Read the model definition and answer for the solid it produces. Units are mm, in the model's axes. A direction names the side the tool comes from. Coordinates: 2 decimals unless noted, no trailing zeros. Loops run counter-clockwise (first coordinate to the right, second up) from the corner with the lowest first, then second, coordinate; pieces in that order, holes last. Notation, with made-up numbers: M 77.5,84 L 98.5,84 A23 cw 98.5,93 Z; hole C 10,21.5 d9. An arc over 180 degrees is marked long. Use one line per item in the form item = value. Start each with the question number.
1. Flat-ended cylindrical pins translate along their axes: pin 1 (1.8 mm diameter, centred on x = -4, y = 0.5, fed in from -Z); pin 2 (2 mm diameter, centred on x = -4.5, y = 18.5, fed in from +Z); pin 3 (1.8 mm diameter, centred on x = -5, z = 7.5, fed in from +Y). Find the tip coordinate at first contact, or state that the pin passes through.
2. For a pull along Y with two mould halves and no side action, classify faces 5 (the flat face through (-4, 1, 11.8)), 6 (the flat face through (-4, -17, 2)), 7 (the cylindrical face through (-6.43, 18.9, 1.83)), 8 (the flat face through (-4, 1, 13.8)) as released by +Y, released by -Y, zero draft, split by the parting line, or undercut.
3. The part is cut by section D-D (x = -2.3). Give the vertices of the cut face in (y, z).
4. A tool of negligible diameter and unlimited length cuts with its end or side. For faces 1 (the flat face through (-4, -11, 6)), 2 (the flat face through (-4, 16, 0.7)), 3 (the flat face through (-4, 16, 3)), 4 (the flat face through (-3, -14, 3)), from which of +Z, -Z, +X, -X, +Y, -Y can it reach the whole face along a straight path? Write none if from no direction.
5. The part is cut by section A-A (y = -15). Give the vertices of the cut face in (x, z).
6. The part is cut by section B-B (z = 4.25). Give the vertices of the cut face in (x, y).
7. The part is cut by section C-C (x = -3.95). Give the vertices of the cut face in (y, z), plus the area to 3 significant figures.
8. Find the intervals of material crossed by probe 1 along X at (y, z) = (17.25, 2.25); probe 2 along Y at (x, z) = (-3.95, 1.8); probe 3 along Y at (x, z) = (-6.2, 4), in increasing order. Write a range as [from, to].
Autodesk Inventor part; units mm, degrees
ref_plane "YZ Plane" through (0, 0, 0) normal (1, 0, 0) x (0, 1, 0)
ref_plane "XZ Plane" through (0, 0, 0) normal (0, 1, 0) x (-1, 0, 0)
ref_plane "XY Plane" through (0, 0, 0) normal (0, 0, 1) x (1, 0, 0)
sketch "Sketch1" plane through (0, 0, 0) normal (0, 0, 1) x (1, 0, 0)
  line L0 (-7, -17) -> (7, -17)
  line L1 (-7, -17) -> (-1, -17)
  line L2 (-1, -17) -> (-1, -11)
  line L3 (-1, -11) -> (-7, -11)
  line L4 (-7, -11) -> (-7, -17)
  line L5 (-5, 19.5) -> (-0.9, 19.5)
  line L6 (-0.9, 19.5) -> (-0.9, 13)
  line L7 (-0.9, 13) -> (-7, 13)
  line L8 (-7, 13) -> (-7, 17.5)
  line L9 (-7, 17.5) -> (-7, -20)
  line L10 (-0.9, 13) -> (-7, 13)
  line L11 (-7, 13) -> (-7, 15)
  line L12 (-7, 15) -> (-0.9, 15)
  line L13 (-0.9, 15) -> (-0.9, 13)
  line L14 (-7, -11) -> (-1, -11)
  line L15 (-1, -11) -> (-1, -13)
  line L16 (-1, -13) -> (-7, -13)
  line L17 (-7, -13) -> (-7, -11)
  circle A0 centre (-3.95, 17.25) radius 0.9
  circle A1 centre (-4, -15) radius 0.9
  arc A2 (-5, 19.5) -> (-7, 17.5) centre (-5, 17.5) ccw
  point P0 (0, 0)
  point P1 (0, 0)
  point P2 (-0.9, 15)
  dimension "d0" = 2
extrude "Extrusion1" add sketch "Sketch1" along normal blind 3 contours L4 L16 L2 L0 | L8 A2 L5 L6 L12
extrude "Extrusion2" add sketch "Sketch1" along normal blind 11.8 contours L8 L12 L6 L7 | L4 L3 L2 L16
sketch "Sketch2" plane through (0, 0, 11.8) normal (0, 0, 1) x (1, 0, 0)
  line L0 (-7, 15) -> (-0.9, 15)
  line L1 (-1, -13) -> (-7, -13)
  line L2 (-0.9, 15) -> (-7, 15)
  line L3 (-7, 15) -> (-7, -13)
  line L4 (-7, -13) -> (-0.9, -13)
  line L5 (-0.9, -13) -> (-0.9, 15)
  point P0 (0, 0)
extrude "Extrusion3" add sketch "Sketch2" along normal blind 2
sketch "Sketch3" plane through (-0.9, 19.5, 3) normal (1, 0, 0) x (0, 0, -1)
  line L0 (3, -6.5) -> (3, 0)
  line L1 (3, 0) -> (0, 0)
  line L2 (0, -4.5) -> (0, 0)
  line L3 (0, -4.5) -> (-10.8, -4.5)
  line L4 (-10.8, -32.5) -> (-10.8, -4.5)
  line L5 (-8.8, -32.5) -> (-10.8, -32.5)
  line L6 (-8.8, -32.5) -> (-8.8, -6.5)
  line L7 (3, -6.5) -> (-8.8, -6.5)
  point P0 (3, -19.5)
extrude "Extrusion4" cut sketch "Sketch3" against normal up to surface (0.1 mm away)
sketch "Sketch4" plane through (0, 0, 0) normal (0, 0, -1) x (-1, 0, 0)
  line L0 (12.228, 25.7128) -> (-5.2106, 25.7128)
  line L1 (-5.2106, 25.7128) -> (-5.2106, -24.037)
  line L2 (-5.2106, -24.037) -> (12.228, -24.037)
  line L3 (12.228, -24.037) -> (12.228, 25.7128)
  point P0 (0, 0)
extrude "Extrusion5" cut sketch "Sketch4" against normal blind 0.7
properties part number "holder servo"
Computed values:
q1.pin_1 = 11.8
q1.pin_2 = 3
q1.pin_3 = 15
q2.face_5 = undercut
q2.face_6 = released by -Y
q2.face_7 = released by +Y
q2.face_8 = zero draft
q3.outline = M -17,0.7 L -11,0.7 L -11,11.8 L 13,11.8 L 13,0.7 L 19.5,0.7 L 19.5,3 L 15,3 L 15,13.8 L -13,13.8 L -13,3 L -17,3 Z
q4.face_1 = -Z, +X, -X
q4.face_2 = -Z, +X, -X, +Y, -Y
q4.face_3 = +Z, +X, -X, +Y
q4.face_4 = +Z, +X, -X, -Y
q5.outline = M -7,0.7 L -4.9,0.7 L -4.9,3 L -7,3 Z; M -3.1,0.7 L -1,0.7 L -1,3 L -3.1,3 Z
q6.outline = M -7,-13 L -1,-13 L -1,-11 L -7,-11 Z; M -7,13 L -1,13 L -1,15 L -7,15 Z
q7.outline = M -17,0.7 L -15.9,0.7 L -15.9,3 L -17,3 Z; M -14.1,0.7 L -11,0.7 L -11,11.8 L 13,11.8 L 13,0.7 L 16.35,0.7 L 16.35,3 L 15,3 L 15,13.8 L -13,13.8 L -13,3 L -14.1,3 Z; M 18.15,0.7 L 19.5,0.7 L 19.5,3 L 18.15,3 Z
q7.area = 112 mm²
q8.probe_1 = [-7, -4.85], [-3.05, -1]
q8.probe_2 = [-17, -15.9], [-14.1, -11], [13, 16.35], [18.15, 19.5]
q8.probe_3 = [-13, -11], [13, 15]
